Design review of the part built by this model. Coordinates are the model's own, in mm. A direction names the side the tool comes from. Give positions to 0.01 mm unless a question says otherwise; leave off trailing zeros. Order: outer loops, then holes, each group sorted by start corner. A loop starts at its lowest first (then second) coordinate and runs counter-clockwise, first axis right, second up. Notation, with made-up numbers: (35.25, 48) -> (49.25, 48) arc R25 cw to (49.25, 83) -> close; hole circle Ø4 at (28.5, 73). An arc over 180 degrees is marked (long way). Answer in a Markdown table with one row per item. Add a question column.
Autodesk Inventor part; units mm, degrees
ref_plane "YZ Plane" through (0, 0, 0) normal (1, 0, 0) x (0, 1, 0)
ref_plane "XZ Plane" through (0, 0, 0) normal (0, 1, 0) x (-1, 0, 0)
ref_plane "XY Plane" through (0, 0, 0) normal (0, 0, 1) x (1, 0, 0)
sketch "Sketch1" plane through (0, 0, 0) normal (0, 0, 1) x (1, 0, 0)
  line L0 (-39.2988, 0) -> (59.8542, 0) construction
  line L1 (0, -36.6223) -> (0, 43.7956) construction
  line L2 (0, 0) -> (32.3074, 32.3074) construction
  line L3 (0, 0) -> (45.6895, 0) construction
  line L4 (0, 24.9041) -> (16.9, 24.9041)
  line L5 (16.9, 24.9041) -> (16.9, 21.2841)
  line L6 (16.9, 21.2841) -> (19.092, 19.092)
  line L7 (24.9041, 0) -> (24.9041, 16.9)
  line L8 (24.9041, 16.9) -> (21.2841, 16.9)
  line L9 (21.2841, 16.9) -> (19.092, 19.092)
  line L10 (0, 24.9041) -> (-16.9, 24.9041)
  line L11 (-16.9, 24.9041) -> (-16.9, 21.2841)
  line L12 (-16.9, 21.2841) -> (-19.092, 19.092)
  line L13 (-24.9041, 0) -> (-24.9041, 16.9)
  line L14 (-24.9041, 16.9) -> (-21.2841, 16.9)
  line L15 (-21.2841, 16.9) -> (-19.092, 19.092)
  line L16 (0, -24.9041) -> (16.9, -24.9041)
  line L17 (16.9, -24.9041) -> (16.9, -21.2841)
  line L18 (16.9, -21.2841) -> (19.092, -19.092)
  line L19 (24.9041, 0) -> (24.9041, -16.9)
  line L20 (24.9041, -16.9) -> (21.2841, -16.9)
  line L21 (21.2841, -16.9) -> (19.092, -19.092)
  line L22 (0, -24.9041) -> (-16.9, -24.9041)
  line L23 (-16.9, -24.9041) -> (-16.9, -21.2841)
  line L24 (-16.9, -21.2841) -> (-19.092, -19.092)
  line L25 (-24.9041, 0) -> (-24.9041, -16.9)
  line L26 (-24.9041, -16.9) -> (-21.2841, -16.9)
  line L27 (-21.2841, -16.9) -> (-19.092, -19.092)
  line L28 (17.13, 25.1341) -> (0, 25.1341)
  line L29 (0, 25.1341) -> (-17.13, 25.1341)
  line L30 (-17.13, 25.1341) -> (-17.13, 21.3793)
  line L31 (-17.13, 21.3793) -> (-19.2547, 19.2547)
  line L32 (-19.2547, 19.2547) -> (-21.3793, 17.13)
  line L33 (-21.3793, 17.13) -> (-25.1341, 17.13)
  line L34 (-25.1341, 17.13) -> (-25.1341, 0)
  line L35 (-25.1341, 0) -> (-25.1341, -17.13)
  line L36 (-25.1341, -17.13) -> (-21.3793, -17.13)
  line L37 (-21.3793, -17.13) -> (-19.2547, -19.2547)
  line L38 (-19.2547, -19.2547) -> (-17.13, -21.3793)
  line L39 (-17.13, -21.3793) -> (-17.13, -25.1341)
  line L40 (-17.13, -25.1341) -> (0, -25.1341)
  line L41 (0, -25.1341) -> (17.13, -25.1341)
  line L42 (17.13, -25.1341) -> (17.13, -21.3793)
  line L43 (17.13, -21.3793) -> (19.2547, -19.2547)
  line L44 (19.2547, -19.2547) -> (21.3793, -17.13)
  line L45 (21.3793, -17.13) -> (25.1341, -17.13)
  line L46 (25.1341, -17.13) -> (25.1341, 0)
  line L47 (25.1341, 0) -> (25.1341, 17.13)
  line L48 (25.1341, 17.13) -> (21.3793, 17.13)
  line L49 (21.3793, 17.13) -> (19.2547, 19.2547)
  line L50 (19.2547, 19.2547) -> (17.13, 21.3793)
  line L51 (17.13, 21.3793) -> (17.13, 25.1341)
  dimension "d27" = 45
  dimension "d28" = 16.9
  dimension "d29" = 3.62
  dimension "d30" = 3.1
  dimension "d31" = 0.23
extrude "Extrusion1" add sketch "Sketch1" along normal blind 5 contours L4 L5 L6 L9 L8 L7 L19 L20 L21 L18 L17 L16 L22 L23 L24 L27 L26 L25 L13 L14 L15 L12 L11 L10 | L51 L50 L49 L48 L47 L46 L45 L44 L43 L42 L41 L40 L39 L38 L37 L36 L35 L34 L33 L32 L31 L30 L29 L28
hole "Hole1" at (0, 0, 0) direction (0, 0, 1) diameter 30 end through all
sketch "Sketch2" plane through (0, 0, 0) normal (0, 0, -1) x (-1, 0, 0)
  circle A0 centre (0, 0) radius 15
  line L0 (3.0701, 14.6825) -> (14.2504, -4.6825)
  line L1 (11.1803, -10) -> (-11.1803, -10)
  line L2 (-14.2504, -4.6825) -> (-3.0701, 14.6825)
  circle A1 centre (0, 0) radius 10 construction
  circle A2 centre (0, 0) radius 15 construction
  circle A3 centre (0, 0) radius 15 construction
  arc A4 (14.2504, -4.6825) -> (3.0701, 14.6825) centre (0, 0) ccw
  arc A5 (-11.1803, -10) -> (11.1803, -10) centre (0, 0) ccw
  arc A6 (-3.0701, 14.6825) -> (-14.2504, -4.6825) centre (0, 0) ccw
  dimension "d22" = 20
extrude "Extrusion2" add sketch "Sketch2" against normal up to surface (5 mm away) contours A0 L0 | L2 A0 | A0 L1
equation "\"Lens_diameter\" = 25"
properties part number "LC_objective_holder"
1) Add section D-D, the plane y = 20. Write out the cut boundary in (x, z), and give its area (3 significant figures).
2) Machinability: for faces 1 (the face through (17.13, 23, 2)), 2 (the face through (23, -17.13, 2)), 3 (the face through (-13.012, -7.463, 2.535)), which of the approach directions +Z, -Z, +X, -X, +Y, -Y give a long, thin tool a straight path to every point of the face, cutting with its end or side? Answer none if there is none.
3) For L1, parallel to Y at x = -23, z = 3.75; L2, parallel to X at y = 14, z = 2.45; L3, parallel to X at y = 0.5, z = 3.45, list the stretches that pass through material, from the lowest coordinate up.
4) Mouldability with a two-part tool opening along Y and no side actions: class faces 4 (the face through (25.134, 0, 2)), 5 (the face through (0, 15, 3)), 6 (the face through (23, 17.13, 2)), 7 (the face through (-23, -17.13, 2)) as +Y half, -Y half, draft (parallel to the pull), parting line (faces both ways), or undercut.
5) Clearance check with flat-ended pins moving along their axes: P1, Ø1.9, axis at y = -22.5, z = 2.5, coming from the +X side; P2, Ø3, axis at y = -23, z = 3.5, coming from the -X side; P3, Ø1.1, axis at x = 22.5, z = 3, coming from the +Y side. State where each tip first meets the part, or that it passes through.
6) Add section B-B, the plane y = -2.5. Write out the cut boundary in (x, z).
7) Add section C-C, the plane z = 3.4. Write out the cut boundary in (x, y).
8) Add section A-A, the plane x = 7. Write out the cut boundary in (y, z).
Verdict:
| question | item | result |
|---|---|---|
| 1 | outline | (-18.51, 0) -> (18.51, 0) -> (18.51, 5) -> (-18.51, 5) -> close |
| 1 | area | 185 mm2 |
| 2 | face 1 | +Z, -Z, +X, +Y |
| 2 | face 2 | +Z, -Z, +X, -Y |
| 2 | face 3 | +Z, -Z |
| 3 | L1 | y = -17.13 to 17.13 |
| 3 | L2 | x = -25.13 to -3.46, 3.46 to 25.13 |
| 3 | L3 | x = -25.13 to -11.26, 11.26 to 25.13 |
| 4 | face 4 | draft |
| 4 | face 5 | undercut |
| 4 | face 6 | +Y half |
| 4 | face 7 | -Y half |
| 5 | P1 | stops at x = 17.13 |
| 5 | P2 | stops at x = -17.13 |
| 5 | P3 | stops at y = 17.13 |
| 6 | outline | (-25.13, 0) -> (-12.99, 0) -> (-12.99, 5) -> (-25.13, 5) -> close; (12.99, 0) -> (25.13, 0) -> (25.13, 5) -> (12.99, 5) -> close |
| 7 | outline | (-25.13, -17.13) -> (-21.38, -17.13) -> (-19.25, -19.25) -> (-17.13, -21.38) -> (-17.13, -25.13) -> (17.13, -25.13) -> (17.13, -21.38) -> (19.25, -19.25) -> (21.38, -17.13) -> (25.13, -17.13) -> (25.13, 17.13) -> (21.38, 17.13) -> (19.25, 19.25) -> (17.13, 21.38) -> (17.13, 25.13) -> (-17.13, 25.13) -> (-17.13, 21.38) -> (-19.25, 19.25) -> (-21.38, 17.13) -> (-25.13, 17.13) -> close; hole (-14.25, -4.68) arc R15 ccw to (-11.18, -10) -> (11.18, -10) arc R15 ccw to (14.25, -4.68) -> (3.07, 14.68) arc R15 ccw to (-3.07, 14.68) -> close |
| 8 | outline | (-25.13, 0) -> (-10, 0) -> (-10, 5) -> (-25.13, 5) -> close; (7.88, 0) -> (25.13, 0) -> (25.13, 5) -> (7.88, 5) -> close |
